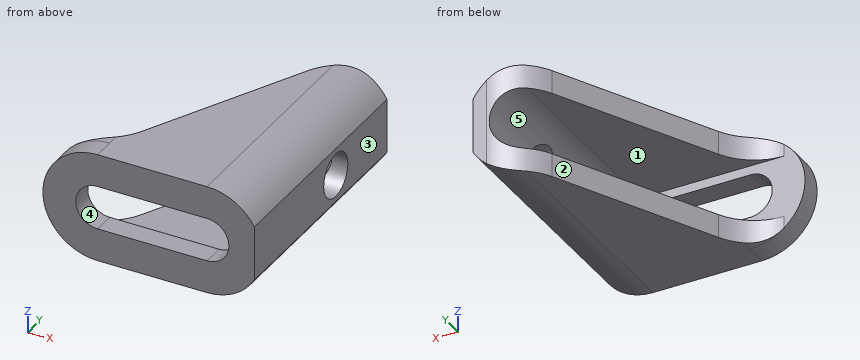
```python
from build123d import *

# Parameters (mm, degrees)
BOSS_EXTRUDE1_DEPTH = 2
SKETCH2_W           = 10
SKETCH2_H           = 2.15
BOSS_EXTRUDE2_DEPTH = 20
CUT_EXTRUDE1_DEPTH  = 29.442925307
FILLET1_START       = -6
FILLET1_DEPTH       = 12
FILLET1_START_2     = 2.85
FILLET1_2_DEPTH     = 1.775923077
FILLET1_START_3     = -4.604846154
FILLET1_3_DEPTH     = 1.754846154
FILLET1_START_4     = -5
FILLET1_4_DEPTH     = 0.395153846
FILLET1_START_5     = 4.625923077
FILLET1_5_DEPTH     = 0.374076923
FILLET1_START_6     = 2
FILLET1_6_DEPTH     = 2.763932023
CUT_EXTRUDE2_DEPTH  = 28.092434523
SKETCH5_R           = 2
CUT_EXTRUDE3_DEPTH  = 30.709490335


with BuildPart() as part:
    # Sketch1 → Boss-Extrude1 (new body)
    with BuildSketch(Plane(origin=(0, 0, 0), x_dir=(1, 0, 0), z_dir=(0, 1, 0))):
        with BuildLine():
            Line((0, 5), (10, 5))
            ThreePointArc((10, 5), (15, 0), (10, -5))
            Line((10, -5), (0, -5))
            ThreePointArc((0, -5), (-5, 0), (0, 5))
        make_face()
        with BuildLine():
            Line((0, 2), (10, 2))
            ThreePointArc((10, 2), (12, 0), (10, -2))
            Line((10, -2), (0, -2))
            ThreePointArc((0, -2), (-2, 0), (0, 2))
        make_face(mode=Mode.SUBTRACT)
    extrude(amount=BOSS_EXTRUDE1_DEPTH)

    # Sketch2 → Boss-Extrude2 (add)
    with BuildSketch(Plane(origin=(0, 2, 0), x_dir=(1, 0, 0), z_dir=(0, 1, 0))):
        with BuildLine():
            ThreePointArc((10, -2.85), (12.85, 0), (10, 2.85))
            Line((10, 2.85), (10, 5))
            ThreePointArc((10, 5), (15, 0), (10, -5))
            Line((10, -5), (10, -2.85))
        make_face()
        with Locations((5, 3.925)):
            Rectangle(SKETCH2_W, SKETCH2_H)
        with Locations((5, -3.925)):
            Rectangle(SKETCH2_W, SKETCH2_H)
    extrude(amount=BOSS_EXTRUDE2_DEPTH)

    # Sketch3 → Cut-Extrude1 (cut, through all)
    with BuildSketch(Plane(origin=(0, 0, -5), x_dir=(-1, 0, 0), z_dir=(0, 0, -1))):
        Polygon((0, 2), (-10, 22), (0, 22), align=None)
    extrude(amount=-CUT_EXTRUDE1_DEPTH, mode=Mode.SUBTRACT)

    # Fillet1: read off the stored shape, not the designer's step
    # Fillet1 outline → Fillet1 (cut)
    with BuildSketch(Plane.XY.offset(FILLET1_START)):
        with BuildLine():
            ThreePointArc((8.618033989, 19.236067977), (10.461514383, 21.253254042), (13.090169944, 22))
            Line((13.090169944, 22), (10, 22))
            Line((10, 22), (8.618033989, 19.236067977))
        make_face()
    extrude(amount=FILLET1_DEPTH, mode=Mode.SUBTRACT)

    # Fillet1 2 outline → Fillet1 2 (add)
    with BuildSketch(Plane.XY.offset(FILLET1_START_2)):
        with BuildLine():
            Line((0, 2), (1.381966011, 4.763932023))
            ThreePointArc((1.381966011, 4.763932023), (-0.461514383, 2.746745958), (-3.090169944, 2))
            Line((-3.090169944, 2), (0, 2))
        make_face()
    extrude(amount=FILLET1_2_DEPTH)

    # Fillet1 3 outline → Fillet1 3 (add)
    with BuildSketch(Plane.XY.offset(FILLET1_START_3)):
        with BuildLine():
            Line((0, 2), (1.381966011, 4.763932023))
            ThreePointArc((1.381966011, 4.763932023), (-0.461514383, 2.746745958), (-3.090169944, 2))
            Line((-3.090169944, 2), (0, 2))
        make_face()
    extrude(amount=FILLET1_3_DEPTH)

    # Fillet1 4 outline → Fillet1 4 (add)
    with BuildSketch(Plane.XY.offset(FILLET1_START_4)):
        with BuildLine():
            Line((0, 2), (1.381966011, 4.763932023))
            ThreePointArc((1.381966011, 4.763932023), (-0.461514383, 2.746745958), (-3.090169944, 2))
            Line((-3.090169944, 2), (0, 2))
        make_face()
    extrude(amount=FILLET1_4_DEPTH)

    # Fillet1 5 outline → Fillet1 5 (add)
    with BuildSketch(Plane.XY.offset(FILLET1_START_5)):
        with BuildLine():
            Line((0, 2), (1.381966011, 4.763932023))
            ThreePointArc((1.381966011, 4.763932023), (-0.461514383, 2.746745958), (-3.090169944, 2))
            Line((-3.090169944, 2), (0, 2))
        make_face()
    extrude(amount=FILLET1_5_DEPTH)

    # Fillet1 6 outline → Fillet1 6 (cut)
    with BuildSketch(Plane(origin=(0, 0, 0), x_dir=(1, 0, 0), z_dir=(0, 1, 0)).offset(FILLET1_START_6)):
        with BuildLine():
            Line((-5, -5), (0, -5))
            ThreePointArc((0, -5), (-3.535533906, -3.535533906), (-5, 0))
            Line((-5, 0), (-5, -5))
        make_face()
        with BuildLine():
            Line((-5, 5), (-5, 0))
            ThreePointArc((-5, 0), (-3.535533906, 3.535533906), (0, 5))
            Line((0, 5), (-5, 5))
        make_face()
    extrude(amount=FILLET1_6_DEPTH, mode=Mode.SUBTRACT)

    # Sketch4 → Cut-Extrude2 (cut, through all)
    with BuildSketch(Plane.XZ):
        with BuildLine():
            Line((14.330127019, 2.5), (14.330127019, -2.5))
            ThreePointArc((14.330127019, -2.5), (15, 0), (14.330127019, 2.5))
        make_face()
    extrude(amount=-CUT_EXTRUDE2_DEPTH, mode=Mode.SUBTRACT)

    # Sketch5 → Cut-Extrude3 (cut, through all)
    with BuildSketch(Plane(origin=(14.330127019, 0, 0), x_dir=(0, 0, -1), z_dir=(1, 0, 0))):
        with Locations((0, 13.5)):
            Circle(SKETCH5_R)
    extrude(amount=-CUT_EXTRUDE3_DEPTH, mode=Mode.SUBTRACT)


solid = part.part
```
Design review of the part built by this model. Coordinates are the model's own, in mm. Face numbers are marked on the shaded views. A direction names the side the tool comes from. Coordinates: 2 decimals unless noted, no trailing zeros. Order: outer loops, then holes, each group sorted by start corner. A loop starts at its lowest first (then second) coordinate and runs counter-clockwise, first axis right, second up. Notation, with made-up numbers: (43.25, -26) -> (77.25, -26) arc R33 ccw to (77.25, 7) -> close; hole circle Ø4 at (63, -29). An arc over 180 degrees is marked (long way). One line per item, written item: value. Start each with the question number.
Q1. Insertion check: pin 1 Ø4 at (x, z) = (-1.5, -3.5) entering from +Y; pin 2 Ø4 at (y, z) = (16.5, 1.5) entering from -X; pin 3 Ø6.5 at (x, y) = (2, 15) entering from +Z; pin 4 Ø5 at (y, z) = (15, 3) entering from -X. Each pin has a flat end and moves straight along its axis. Give the tip position at first contact, or say it passes through.
Q2. Take a section at D-D, the plane x = 4.75. State the section outline as (y, z) points.
Q3. Tool access review of the marked faces 1 and 2: name each direction out of +Z, -Z, +X, -X, +Y, -Y from which nothing blocks a thin tool from reaching the whole face with its end or side.
Q4. Take a section at C-C, the plane z = 0. State the section outline as (x, y) points.
Q5. Mouldability with a two-part tool opening along X and no side actions: class the marked faces 3, 4 and 5 as pulls with the +X half, pulls with the -X half, needs draft (parallel to the pull), parting line crosses it, or undercut.
Q6. Take a section at B-B, the plane y = 13.5. State the section outline as (x, z) points, then the cut area to 3 significant figures.
Q7. For probe 1 along Z at (x, y) = (9.75, 11); probe 2 along Y at (x, z) = (13.15, 0); probe 3 along X at (y, z) = (4.75, 2), list the stretches that pass through material, from the lowest coordinate up.
Q8. Take a section at A-A, the plane x = 8.25. State the section outline as (y, z) points.
Values follow:
1. pin 1: stops at y = 3.52
1. pin 2: stops at x = 6.51
1. pin 3: passes through
1. pin 4: stops at x = 5.25
2. outline: (0, -5) -> (11.5, -5) -> (11.5, -2.85) -> (2, -2.85) -> (2, -2) -> (0, -2) -> close; (0, 2) -> (2, 2) -> (2, 2.85) -> (11.5, 2.85) -> (11.5, 5) -> (0, 5) -> close
3. face 1: -X, +Y
3. face 2: +Z, -Z, -X, +Y
4. outline: (-5, 0) -> (-2, 0) -> (-2, 2) -> (-5, 2) -> close; (12, 0) -> (14.33, 0) -> (14.33, 11.5) -> (12.85, 11.5) -> (12.85, 2) -> (12, 2) -> close; (12.85, 15.5) -> (14.33, 15.5) -> (14.33, 22) -> (13.09, 22) arc R5 ccw to (12.85, 21.99) -> close
5. face 3: pulls with the +X half
5. face 4: undercut
5. face 5: pulls with the -X half
6. outline: (5.75, -5) -> (10, -5) arc R5 ccw to (14.33, -2.5) -> (14.33, -2) -> (12.03, -2) arc R2.85 cw to (10, -2.85) -> (5.75, -2.85) -> close; (5.75, 2.85) -> (10, 2.85) arc R2.85 cw to (12.03, 2) -> (14.33, 2) -> (14.33, 2.5) arc R5 ccw to (10, 5) -> (5.75, 5) -> close
6. area: 35.6 mm2
7. probe 1: z = -5 to -2.85, 2.85 to 5
7. probe 2: y = 0 to 11.5, 15.5 to 22
7. probe 3: x = 12.03 to 14.33
8. outline: (0, -5) -> (18.5, -5) -> (18.5, -2.85) -> (2, -2.85) -> (2, -2) -> (0, -2) -> close; (0, 2) -> (2, 2) -> (2, 2.85) -> (18.5, 2.85) -> (18.5, 5) -> (0, 5) -> close
